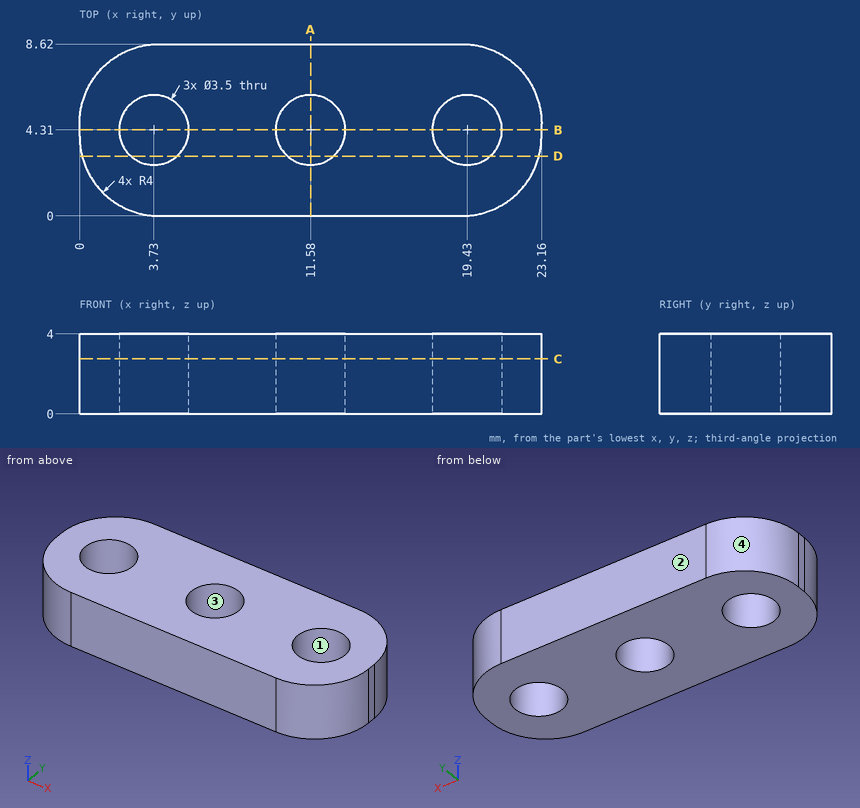
Job drawing, mm, ordinate dimensions from the low corner. One solid piece. Give positions to 0.01 mm unless a question says otherwise; leave off trailing zeros. Order: outer loops, then holes, each group sorted by start corner. A loop starts at its lowest first (then second) coordinate and runs counter-clockwise, first axis right, second up. Notation, with made-up numbers: (78, -6) - (91, -6) arc R24 ccw to (91, 7) - close; hole circle Ø9 at (30, 2). An arc over 180 degrees is marked (long way). Return JSON: item names as keys, results as strings.
1) Probe line 1 (Y direction, x = 11.58, z = 2.05); line 2 (X direction, y = 5.75, z = 1.1); line 3 (X direction, y = 3.75, z = 3.3). List the from-to ranges inside material, lowest first. Write a range as from..to.
Geometry says:
{"line 1": "0..2.56, 6.06..8.62", "line 2": "0.16..2.74, 4.72..10.59, 12.57..18.44, 20.42..23", "line 3": "0.01..2.07, 5.39..9.92, 13.24..17.77, 21.09..23.15"}
2) Cut at C-C, the plane z = 2.75. Give the cut face in (x, y), plus the area to 3 significant figures.
Geometry says:
{"outline": "(0, 4) arc R4 ccw to (4, 0) - (19.16, 0) arc R4 ccw to (23.16, 4) - (23.16, 4.62) arc R4 ccw to (19.16, 8.62) - (4, 8.62) arc R4 ccw to (0, 4.62) - close; hole circle Ø3.5 at (3.73, 4.31); hole circle Ø3.5 at (11.58, 4.31); hole circle Ø3.5 at (19.43, 4.31)", "area": "157 mm²"}
3) Cut at D-D, the plane y = 3. Give the cut face in (x, z).
Geometry says:
{"outline": "(0.13, 0) - (2.57, 0) - (2.57, 4) - (0.13, 4) - close; (4.89, 0) - (10.42, 0) - (10.42, 4) - (4.89, 4) - close; (12.74, 0) - (18.27, 0) - (18.27, 4) - (12.74, 4) - close; (20.59, 0) - (23.03, 0) - (23.03, 4) - (20.59, 4) - close"}
4) Cut at A-A, the plane x = 11.58. Give the cut face in (y, z), plus the area to 3 significant figures.
Geometry says:
{"outline": "(0, 0) - (2.56, 0) - (2.56, 4) - (0, 4) - close; (6.06, 0) - (8.62, 0) - (8.62, 4) - (6.06, 4) - close", "area": "20.5 mm²"}
5) Pull direction X, two halves, no side cores. Call the marked faces 1, 2, 3 and 4: pulls with the +X half, pulls with the -X half, needs draft (parallel to the pull), parting line crosses it, or undercut.
Geometry says:
{"face 1": "undercut", "face 2": "needs draft", "face 3": "undercut", "face 4": "pulls with the -X half"}
6) Cut at B-B, the plane y = 4.31. Give the cut face in (x, z), plus the area to 3 significant figures.
Geometry says:
{"outline": "(0, 0) - (1.98, 0) - (1.98, 4) - (0, 4) - close; (5.48, 0) - (9.83, 0) - (9.83, 4) - (5.48, 4) - close; (13.33, 0) - (17.68, 0) - (17.68, 4) - (13.33, 4) - close; (21.18, 0) - (23.16, 0) - (23.16, 4) - (21.18, 4) - close", "area": "50.6 mm²"}
7) Flat gauge pins, fed straight in: P1, Ø2, axis at y = 1.5, z = 0.5, coming from the +X side; P2, Ø3, axis at x = 11.58, y = 4.31, coming from the +Z side; P3, Ø2, axis at x = 2.5, z = 2.5, coming from the +Y side. Where does each tip first touch, or does it go through?
Geometry says:
{"P1": "x = 22.87", "P2": "through", "P3": "y = 8.59"}
